Input: part model. Units: mm. Frame: model coordinates. A direction names the side the tool comes from. Coordinates: 2 decimals unless noted, no trailing zeros. Loops run counter-clockwise (first coordinate to the right, second up) from the corner with the lowest first, then second, coordinate; pieces in that order, holes last. Notation, with made-up numbers: (17, 3.25) -> (52, 3.25) arc R20 cw to (52, 22.25) -> close; hole circle Ø2 at (86, 76.5). An arc over 180 degrees is marked (long way). Put each result on its own line as item: value. Start each with the question number.
1) Material intervals for L1, parallel to X at y = -4.25, z = -4; L2, parallel to X at y = 5.5, z = -5; L3, parallel to Z at x = 12.5, y = 3, sorted ascending.
2) Set-up query: faces 1 (the flat face through (-3.46, -6.961, -3.944)), 2 (the flat face through (-0.6, -7, -3)). Return all of +Z, -Z, +X, -X, +Y, -Y with unobstructed straight access to the full face (end or side cutting, diameter ignored); none if empty.
3) Contact query for flat-ended pins moving along their axis: P1, Ø1, axis at x = 21.5, y = 6.5, coming from the -Z side; P2, Ø8, axis at x = 24, y = 7, coming from the +Z side; P3, Ø3, axis at y = 6.5, z = -3, coming from the +X side; P4, Ø2, axis at x = 9.5, y = 3, coming from the -Z side. Output: stop coordinate, or through.
4) Cut plane A-A (x = 26.5). Return the cut outline in (y, z).
Autodesk Inventor part; units mm, degrees
ref_plane "Work Plane1" through (1.525, 0, 0) normal (0, 0, 1) x (1, 0, 0)
ref_plane "YZ Plane" through (0, 0, 0) normal (1, 0, 0) x (0, 1, 0)
ref_plane "XZ Plane" through (0, 0, 0) normal (0, 1, 0) x (-1, 0, 0)
sketch "Sketch1" plane through (0, 0, 0) normal (0, 0, 1) x (1, 0, 0)
  line L0 (0, 7.315) -> (0, 5)
  line L1 (4, 5) -> (30, 5)
  line L2 (30, 5) -> (30, 0)
  line L3 (30, 0) -> (-0.6001, 0)
  line L4 (-6.7201, 0) -> (36.12, 0)
  line L5 (-0.6001, 0) -> (-0.6001, 7.315)
  line L6 (-0.6001, 7.315) -> (0, 7.315)
  line L7 (4, 5) -> (3.0797, 5)
  line L8 (3.0797, 5) -> (0, 5)
  line L9 (0, -1.463) -> (0, 8.778)
  dimension "d0" = 30
  dimension "d1" = 26
  dimension "d2" = 10
  dimension "d9" = 0.6001
  dimension "d10" = 14.63
  dimension "d13" = 0.9203
  dimension "d14" = 10
revolve "Body" add sketch "Sketch1" angle 360 about axis through (30, 0, 0) along (-1, 0, 0)
sketch "Sketch2" plane through (-0.6001, 0, 0) normal (-1, 0, 0) x (0, 0, 1)
  line L0 (0, 9.2376) -> (8, 4.6188)
  line L1 (8, 4.6188) -> (8, -4.6188)
  line L2 (8, -4.6188) -> (0, -9.2376)
  line L3 (0, -9.2376) -> (-8, -4.6188)
  line L4 (-8, -4.6188) -> (-8, 4.6188)
  line L5 (-8, 4.6188) -> (0, 9.2376)
  point P0 (0, 0)
  point P1 (0, 0)
  dimension "d11" = 16
extrude "Head" add sketch "Sketch2" along normal blind 5.8
sketch "Sketch4" plane through (0, 0, 0) normal (0, 0, 1) x (1, 0, 0)
  line L0 (-6.4001, 8) -> (-6.4001, 9.2376)
  line L1 (-6.4001, 9.2376) -> (-5.6856, 9.2376)
  line L2 (-5.6856, 9.2376) -> (-6.4001, 8)
  line L3 (-7.5601, 0) -> (0.5599, 0)
  line L4 (-0.6001, 9.2376) -> (-6.4001, 9.2376)
  line L5 (-6.4001, 4.6188) -> (-6.4001, 9.2376)
  dimension "d5" = 30
  dimension "d19" = 16
revolve "Chamfer1" cut sketch "Sketch4" angle 360 about axis through (-10, 0, 0) along (1, 0, 0)
thread "Thread"
chamfer "Chamfer2" distance 0.9202 distance2 0.9203 1 edges at (30, -5, 0) measured on face at (30, -0.2009, 0.1054)
ref_plane "Work Plane1" through (1.525, 0, 0) normal (0, 0, 1) x (1, 0, 0)
equation "\"d11\" = SW"
equation "\"d3\" = KOH - SD"
equation "\"d15\" = GD"
equation "\"d6\" = -0.5 * SPD + 0.5 * GD"
equation "\"d1\" = GEL"
equation "\"d2\" = GD"
equation "\"d10\" = SD2"
equation "\"d14\" = BDM"
equation "\"d5\" = ANG1"
equation "\"d19\" = SW0"
equation "\"NLG\" = 45"
equation "\"GD\" = NND"
equation "\"BDM\" = NND"
equation "\"KOH\" = 6.4"
equation "\"GEL\" = 26"
equation "\"SW\" = 16"
equation "\"SW0\" = SW"
equation "\"SPD\" = NND - 1.2269 * PTC"
equation "\"SD2\" = 14.63"
equation "\"SD\" = 0.6"
equation "\"ANG1\" = 30deg"
equation "\"GAL\" = 0.61345 * PTC"
equation "\"GUL\" = 0.61345 * PTC"
equation "\"RR\" = 0.4"
equation "\"GD1\" = THREADDIA - 1.2269 * PTC"
equation "\"SDH\" = SD2"
equation "\"TOA\" = 30deg"
equation "\"PTC\" = 1.5"
equation "\"E0\" = 1.155 * SW"
properties part number "ISO 4014 - M10 x 45" material "Stainless Steel, 440C"
Results found:
1. L1: x = -6.4 to 0
1. L2: x = -6.4 to -0.6
1. L3: z = -4 to 4
2. face 1: -Z, +X, -X, -Y
2. face 2: +X
3. P1: passes through
3. P2: stops at z = 4
3. P3: stops at x = 0
3. P4: stops at z = -4.58
4. outline: circle Ø10 at (0, 0)
